```python
from build123d import *

# Parameters (mm, degrees)
F0_W     = 150
F0_H     = 79.84
F0_R     = 3.25
F0_R_2   = 1
F0_R_3   = 2.75
F0_R_4   = 7.5
F0_R_5   = 14.5
F1_DEPTH = 8
F2_SIZE  = 3
F4_D     = 3.3


with BuildPart() as f1:
    # F0 (on Top) → F1 (new body)
    with BuildSketch(Plane.XY):
        with Locations((0, 0.08)):
            Rectangle(F0_W, F0_H)
        with Locations((-66.8569050639, -32.9713009074)):
            Circle(F0_R, mode=Mode.SUBTRACT)
        with Locations((-41.9708455764, -4.2951276581)):
            Circle(F0_R_2, mode=Mode.SUBTRACT)
        with Locations((-8.25, -8.25)):
            Circle(F0_R_3, mode=Mode.SUBTRACT)
        with Locations((68.1422611349, -32.4968268505)):
            Circle(F0_R, mode=Mode.SUBTRACT)
        with Locations((8.25, -8.25)):
            Circle(F0_R_3, mode=Mode.SUBTRACT)
        Circle(F0_R_4, mode=Mode.SUBTRACT)
        with Locations((42, -4)):
            Circle(F0_R_2, mode=Mode.SUBTRACT)
        with Locations((-61.1039310143, 14.5708481086)):
            Circle(F0_R_2, mode=Mode.SUBTRACT)
        with Locations((-42.104400412, 14.7044029442)):
            Circle(F0_R_5, mode=Mode.SUBTRACT)
        with Locations((-8.25, 8.25)):
            Circle(F0_R_3, mode=Mode.SUBTRACT)
        with Locations((-23.1048698098, 14.8379577797)):
            Circle(F0_R_2, mode=Mode.SUBTRACT)
        with Locations((-67.4991661988, 32.0255259431)):
            Circle(F0_R, mode=Mode.SUBTRACT)
        with Locations((-42.2379552476, 33.7039335464)):
            Circle(F0_R_2, mode=Mode.SUBTRACT)
        with Locations((8.25, 8.25)):
            Circle(F0_R_3, mode=Mode.SUBTRACT)
        with Locations((23, 15)):
            Circle(F0_R_2, mode=Mode.SUBTRACT)
        with Locations((42, 15)):
            Circle(F0_R_5, mode=Mode.SUBTRACT)
        with Locations((61, 15)):
            Circle(F0_R_2, mode=Mode.SUBTRACT)
        with Locations((42, 34)):
            Circle(F0_R_2, mode=Mode.SUBTRACT)
        with Locations((67.5, 32.5)):
            Circle(F0_R, mode=Mode.SUBTRACT)
    extrude(amount=F1_DEPTH)

    # F2
    f2_edges = [f1.edges().sort_by_distance(p)[0] for p in [
        (75, -39.84, 4),
        (75, 40, 4),
        (-75, -39.84, 4),
        (-75, 40, 4),
    ]]
    chamfer(f2_edges, length=F2_SIZE)

    # F4 (through all)
    with Locations(Plane.XY.offset(8)):
        with Locations((42, 34), (61, 15), (42, -4), (23, 15), (-23.1048698098, 14.8379577797), (-42.2379552476, 33.7039335464), (-41.9708455764, -4.2951276581), (-61.1039310143, 14.5708481086)):
            Hole(F4_D / 2)


solid = f1.part
```
Check sheet for the modelled part. Datum: model origin and axes. Units: mm. Round coordinates to 2 decimals unless told otherwise and drop trailing zeros. Loops run counter-clockwise (first coordinate to the right, second up) from the corner with the lowest first, then second, coordinate; pieces in that order, holes last. Notation, with made-up numbers: (50, 19) - (92, 19) arc R4 ccw to (92, 25) - close; hole circle Ø1 at (48.5, 53.25). An arc over 180 degrees is marked (long way). Write item = value, one per line. Start each with the question number.
Q1. Section check A-A (x = 23). Record the boundary of the cut face in (y, z), plus the area to 3 significant figures.
Q2. Depth check by flat-ended pin: P1, Ø9, axis at x = 8.25, y = -8.25, coming from the -Z side; P2, Ø2, axis at x = -23.1, y = 14.84, coming from the -Z side. Enter the tip coordinate at first touch or a pass-through.
Q3. Thickness scan on L1, parallel to Y at x = 42, z = 3.5; L2, parallel to Y at x = -8.25, z = 4.25; L3, parallel to X at y = -30.5, z = 6.25. Record the ranges inside material, lowest first.
Q4. Release check for a two-part mould opening along X. For faces 1 (the face through (-1, -8, 8)), 2 (the face through (-65.11, -30.23, 3.94)), 3 (the face through (73.52, -38.32, 3.94)) record: pulls with the +X half, pulls with the -X half, needs draft (parallel to the pull), parting line crosses it, or undercut.
Q5. Section check D-D (x = 67.5). Record the boundary of the cut face in (y, z), plus the area to 3 significant figures.
Q6. Section check C-C (z = 3). Count the separate pieces of the cut face and the enclosed holes in it, plus the area to 3 significant figures.
Q7. Section check B-B (y = 21.5). Record the boundary of the cut face in (x, z).
Derived:
q1.outline = (-39.84, 0) - (13.35, 0) - (13.35, 8) - (-39.84, 8) - close; (16.65, 0) - (40, 0) - (40, 8) - (16.65, 8) - close
q1.area = 612 mm^2
q2.P1 = 0
q2.P2 = through
q3.L1 = -39.84 to -5.65, -2.35 to 0.5, 29.5 to 32.35, 35.65 to 40
q3.L2 = -39.84 to -11, -5.5 to 5.5, 11 to 40
q3.L3 = -75 to -68.97, -64.75 to 65.58, 70.71 to 75
q4.face_1 = needs draft
q4.face_2 = undercut
q4.face_3 = pulls with the +X half
q5.outline = (-39.84, 0) - (-35.68, 0) - (-35.68, 8) - (-39.84, 8) - close; (-29.31, 0) - (29.25, 0) - (29.25, 8) - (-29.31, 8) - close; (35.75, 0) - (40, 0) - (40, 8) - (35.75, 8) - close
q5.area = 536 mm^2
q6.separate_pieces = 1
q6.enclosed_holes = 19
q6.area = 10,200 mm^2
q7.outline = (-75, 0) - (-54.91, 0) - (-54.91, 8) - (-75, 8) - close; (-29.3, 0) - (29.04, 0) - (29.04, 8) - (-29.3, 8) - close; (54.96, 0) - (75, 0) - (75, 8) - (54.96, 8) - close
